Verification items for the finished model (mm, model axes). A direction names the side the tool comes from. Coordinates: 2 decimals unless noted, no trailing zeros. Order: outer loops, then holes, each group sorted by start corner. A loop starts at its lowest first (then second) coordinate and runs counter-clockwise, first axis right, second up.
Q1. Cross-section at A-A, the plane z = -7. Record the boundary of the cut face in (x, y).
Q2. Set-up check for faces 4 (the cylindrical face through (-11.99, -0.53, -10.14)), 5 (the cylindrical face through (-14.985, -0.66, -9.86)): record each of +Z, -Z, +X, -X, +Y, -Y from which the full face is reachable in a straight line by a thin tool's end or side.
Q3. Thickness scan on line 1 (X direction, y = 0, z = -20); line 2 (X direction, y = 0, z = -4). Record the ranges inside material, lowest first.
Q4. Draft check along Y on faces 1 (the cylindrical face through (-6, 0, -23)), 2 (the flat face through (-7, -10, 0)), 3 (the cylindrical face through (2.82, 5.43, -31.6)). Enter one of: pulls with the +Y half, pulls with the -Y half, needs draft (parallel to the pull), parting line crosses it, or undercut.
Q5. Depth check by flat-ended pin: P1, Ø5, axis at x = -6.5, y = -10, coming from the -Z side; P2, Ø2, axis at y = 4.5, z = -27.5, coming from the +X side; P3, Ø12, axis at y = -7.5, z = -21.5, coming from the +X side. Enter the tip coordinate at first touch or a pass-through.
from build123d import *


# Not quite as in the source:
# - a fillet or chamfer that OpenCascade refuses, or shapes differently, is made with other operations: its cross-section is extruded or revolved along the edge and cut away or added


with BuildPart() as f1:
    # F0 (on Front) → F1 (revolve)
    with BuildSketch(Plane.XZ):
        with BuildLine():
            Line((15, 0), (13.5, 0))
            Line((13.5, 0), (12, 0))
            Line((12, 0), (12, -1.5))
            Line((12, -1.5), (12, -20))
            ThreePointArc((12, -20), (10.3452954698, -25.1406164595), (6, -28.3472333599))
            ThreePointArc((6, -28.3472333599), (5.0122671395, -28.6160728483), (4, -28.7684083747))
            Line((4, -28.7684083747), (4, -31.7684083747))
            Line((4, -31.7684083747), (6.1201079457, -31.7684083747))
            Line((6.1201079457, -31.7684083747), (6.1201079457, -31.4292851344))
            ThreePointArc((6.1201079457, -31.4292851344), (12.5191285439, -27.2367299518), (15, -20))
            Line((15, -20), (15, 0))
        make_face()
        with BuildLine():
            ThreePointArc((4, -28.7684083747), (5.0122671395, -28.6160728483), (6, -28.3472333599))
            Line((6, -28.3472333599), (6, -13.7684083747))
            Line((6, -13.7684083747), (4, -13.7684083747))
            Line((4, -13.7684083747), (4, -28.7684083747))
        make_face()
    revolve(axis=Axis((0, 0, -27.0683728158), (0, 0, -1)))

    # F2: fillet of radius 5 on 1 edges, made by hand

    # F2_s1 → F2_t2 (revolve, cut)
    with BuildSketch(Plane.XZ):
        with BuildLine():
            ThreePointArc((6, -17.7684083747), (5.472135955, -15.5323403972), (4, -13.7684083747))
            Line((4, -13.7684083747), (6, -13.7684083747))
            Line((6, -13.7684083747), (6, -17.7684083747))
        make_face()
    revolve(axis=Axis((0, 0, -13.7684083747), (0, 0, -1)), mode=Mode.SUBTRACT)


solid = f1.part
Check values:
1. outline: circle Ø30 at (0, 0); hole circle Ø24 at (0, 0)
2. face 4: +Z
2. face 5: +Z, -Z
3. line 1: x = -15 to -12, -6 to -4, 4 to 6, 12 to 15
3. line 2: x = -15 to -12, 12 to 15
4. face 1: undercut
4. face 2: needs draft
4. face 3: parting line crosses it
5. P1: stops at z = -30.02
5. P2: stops at x = 12.33
5. P3: stops at x = 14.91
